Source: three-view drawing plus pictorial views. Frame: mm from the lowest corner of the part. A direction names the side the tool comes from. Give positions to 0.01 mm unless a question says otherwise; leave off trailing zeros. Loops run counter-clockwise (first coordinate to the right, second up) from the corner with the lowest first, then second, coordinate; pieces in that order, holes last.
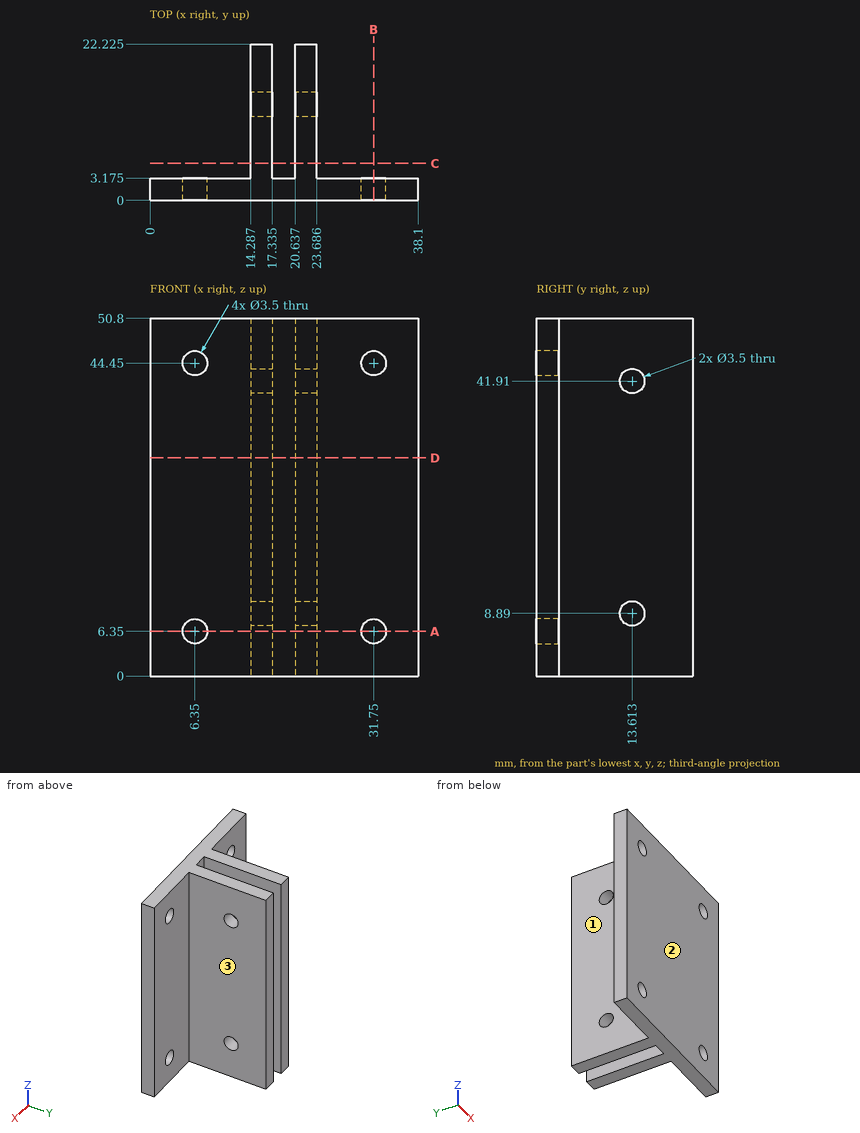
(1) Cut plane B-B (x = 31.75). Return the cut outline in (y, z) (1 decimal), and give its area (3 significant figures).
Values follow:
outline: (0, 0) - (3.2, 0) - (3.2, 4.6) - (0, 4.6) - close; (0, 8.1) - (3.2, 8.1) - (3.2, 42.7) - (0, 42.7) - close; (0, 46.2) - (3.2, 46.2) - (3.2, 50.8) - (0, 50.8) - close
area: 139 mm2
(2) Cut plane C-C (y = 5.25). Return the cut outline in (x, z) (1 decimal).
Values follow:
outline: (14.3, 0) - (17.3, 0) - (17.3, 50.8) - (14.3, 50.8) - close; (20.6, 0) - (23.7, 0) - (23.7, 50.8) - (20.6, 50.8) - close
(3) Pin query (flat end, axial travel): pin 1 Ø9.5 at (y, z) = (10, 14) entering from +X (1 decimal); pin 2 Ø4 at (x, z) = (31.75, 6.35) entering from +Y (1 decimal); pin 3 Ø5.5 at (y, z) = (10, 19) entering from -X. Return the tip coordinate at first contact, or that it passes through.
Values follow:
pin 1: stops at x = 23.7
pin 2: stops at y = 3.2
pin 3: stops at x = 14.29
(4) Cut plane D-D (z = 31). Return the cut outline in (x, y) (1 decimal).
Values follow:
outline: (0, 0) - (38.1, 0) - (38.1, 3.2) - (23.7, 3.2) - (23.7, 22.2) - (20.6, 22.2) - (20.6, 3.2) - (17.3, 3.2) - (17.3, 22.2) - (14.3, 22.2) - (14.3, 3.2) - (0, 3.2) - close
(5) Reachability of the marked faces 1, 2 and 3 from +Z, -Z, +X, -X, +Y, -Y: full face, straight path, thin tool, end or side. Return the list, or none.
Values follow:
face 1: +Z, -Z, -X, +Y
face 2: +Z, -Z, +X, -X, -Y
face 3: +Z, -Z, +X, +Y
(6) Ray query, probe 1 along X at (y, z) = (1.4, 44.45); probe 2 along X at (y, z) = (19.5, 35) (1 decimal); probe 3 along Z at (x, y) = (30.5, 2) (1 decimal). Return the intervals inside material, ascending.
Values follow:
probe 1: x = 0 to 4.6, 8.1 to 30, 33.5 to 38.1
probe 2: x = 14.3 to 17.3, 20.6 to 23.7
probe 3: z = 0 to 5.1, 7.6 to 43.2, 45.7 to 50.8
(7) Cut plane A-A (z = 6.35). Return the cut outline in (x, y) (1 decimal).
Values follow:
outline: (0, 0) - (4.6, 0) - (4.6, 3.2) - (0, 3.2) - close; (8.1, 0) - (30, 0) - (30, 3.2) - (23.7, 3.2) - (23.7, 22.2) - (20.6, 22.2) - (20.6, 3.2) - (17.3, 3.2) - (17.3, 22.2) - (14.3, 22.2) - (14.3, 3.2) - (8.1, 3.2) - close; (33.5, 0) - (38.1, 0) - (38.1, 3.2) - (33.5, 3.2) - close
